For this review, take the finished solid that the model builds, in its own axes (mm). Round coordinates to 2 decimals unless told otherwise and drop trailing zeros. Loops run counter-clockwise (first coordinate to the right, second up) from the corner with the lowest first, then second, coordinate; pieces in that order, holes last. Notation, with made-up numbers: (21, 69.25) -> (44, 69.25) arc R17 ccw to (44, 81.25) -> close; hole circle Ø9 at (60, 57). An arc over 180 degrees is marked (long way). One line per question, with ' | ' between items. Start each with the question number.
1. Consider section D-D (y = -2). Write out the cut boundary in (x, z), and give its area (3 significant figures).
2. Consider section A-A (y = 40). Write out the cut boundary in (x, z).
3. Consider section C-C (x = 3.75). Write out the cut boundary in (y, z).
4. For pin 1 Ø6 at (y, z) = (-7.5, -0.5) entering from -X, flat-tipped, find the tip position at first contact; note if it passes through.
5. Consider section B-B (z = 0). Write out the cut boundary in (x, y).
6. Wall thickness on line 1 along Z through (x, y) = (2.3, 0); line 2 along Y through (x, z) = (3.9, 2.5); line 3 along Z through (x, y) = (4.55, 36): over which ranges is each line inside the solid? List them lowest first.
```python
from build123d import *

# Parameters (mm, degrees)
F0_W     = 100
F0_H     = 60
F0_R     = 7.07
F1_DEPTH = 5


with BuildPart() as f1:
    # F0 (on Right) → F1 (new body)
    with BuildSketch(Plane.YZ):
        with Locations((20, 0)):
            Rectangle(F0_W, F0_H)
        Circle(F0_R, mode=Mode.SUBTRACT)
        with Locations((40, 0)):
            Circle(F0_R, mode=Mode.SUBTRACT)
    extrude(amount=F1_DEPTH)


solid = f1.part
```
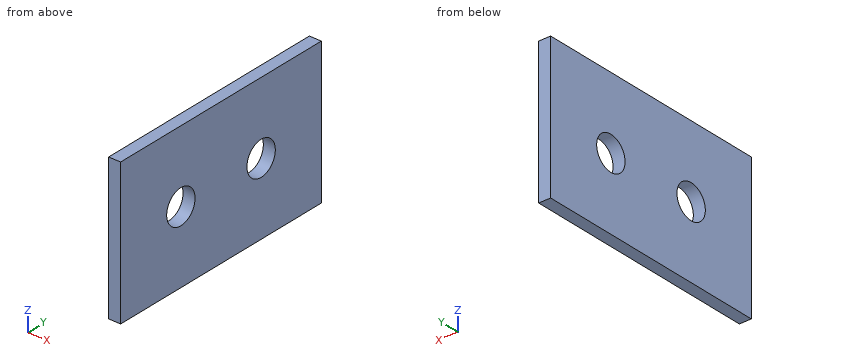
Answer block:
1) outline: (0, -30) -> (5, -30) -> (5, -6.78) -> (0, -6.78) -> close; (0, 6.78) -> (5, 6.78) -> (5, 30) -> (0, 30) -> close | area: 232 mm2
2) outline: (0, -30) -> (5, -30) -> (5, -7.07) -> (0, -7.07) -> close; (0, 7.07) -> (5, 7.07) -> (5, 30) -> (0, 30) -> close
3) outline: (-30, -30) -> (70, -30) -> (70, 30) -> (-30, 30) -> close; hole circle Ø14.14 at (0, 0); hole circle Ø14.14 at (40, 0)
4) pin 1: stops at x = 0
5) outline: (0, -30) -> (5, -30) -> (5, -7.07) -> (0, -7.07) -> close; (0, 7.07) -> (5, 7.07) -> (5, 32.93) -> (0, 32.93) -> close; (0, 47.07) -> (5, 47.07) -> (5, 70) -> (0, 70) -> close
6) line 1: z = -30 to -7.07, 7.07 to 30 | line 2: y = -30 to -6.61, 6.61 to 33.39, 46.61 to 70 | line 3: z = -30 to -5.83, 5.83 to 30
